Check sheet for the modelled part. Datum: model origin and axes. Units: mm. A direction names the side the tool comes from. Round coordinates to 2 decimals unless told otherwise and drop trailing zeros. Loops run counter-clockwise (first coordinate to the right, second up) from the corner with the lowest first, then second, coordinate; pieces in that order, holes last. Notation, with made-up numbers: (27.25, 27) - (41.25, 27) arc R18 cw to (41.25, 41) - close; hole circle Ø3 at (-9, -22.75). An arc over 180 degrees is marked (long way). Answer in a Markdown table with one row per item. Add a question column.
(1) Mould release check, pull along X, two halves, no side actions. Record for faces 3 (the cylindrical face through (10, 8, 2)), 4 (the flat face through (6.9, 2, -0.5)), 5 (the flat face through (14, 15, 2)): +X half, -X half, draft (parallel to the pull), parting line (faces both ways), or undercut.
(2) Gauge pin test, flat end, axial feed: pin 1 (4 mm diameter, centred on x = 6, y = 11, fed in from -Z). Record the tip position at first contact, or that the pin passes through.
(3) Thickness scan on line 1 along X through (y, z) = (12.5, 3.15); line 2 along Y through (x, z) = (7.75, -0.55); line 3 along Z through (x, y) = (6, 8.5). Record the ranges inside material, lowest first.
(4) Access from +Z, -Z, +X, -X, +Y, -Y to the whole of each face (thin tool, end or side, straight path). Record for faces 1 (the flat face through (6.9, 30, 3.5)), 2 (the flat face through (7, 9, 0)).
(5) Cross-section at A-A on y = 6. Enter the section's corners in (x, z), then the cut area to 3 significant figures.
(6) Cross-section at B-B on z = 3.4. Enter the section's corners in (x, y).
(7) Cross-section at C-C on z = 1.9. Enter the section's corners in (x, y).
from build123d import *

# Parameters (mm, degrees)
ESQUISSE1_W                = 14
ESQUISSE1_H                = 30
BASE_EXTRUSION_DEPTH       = 5
ESQUISSE2_W                = 4
ESQUISSE2_H                = 29
ENL_V_MAT_EXTRU_2_DEPTH    = 34.481338086
CONG_2_R                   = 3
ENL_V_MAT_EXTRU_3_DEPTH    = 20
R_P_TITION_LIN_AIRE1_COUNT = 14
R_P_TITION_LIN_AIRE1_PITCH = 1
ESQUISSE10_W               = 2
ESQUISSE10_H               = 3
ENL_V_MAT_EXTRU_17_DEPTH   = 20
ESQUISSE11_W               = 2
ESQUISSE11_H               = 2
BOSS_EXTRU_2_DEPTH         = 14
ESQUISSE12_R               = 2.5
ENL_V_MAT_EXTRU_18_DEPTH   = 34.346664001
ESQUISSE13_R               = 2.1
ENL_V_MAT_EXTRU_19_DEPTH   = 14


with BuildPart() as part:
    # Esquisse1 → Base-Extrusion (new body)
    with BuildSketch(Plane.XY):
        with Locations((7, 15)):
            Rectangle(ESQUISSE1_W, ESQUISSE1_H)
    extrude(amount=BASE_EXTRUSION_DEPTH)

    # Esquisse2 → Enlèv. mat.-Extru.2 (cut, through all)
    with BuildSketch(Plane(origin=(14, 0, 0), x_dir=(0, 0, -1), z_dir=(1, 0, 0))):
        with Locations((-6, 16.5)):
            Rectangle(ESQUISSE2_W, ESQUISSE2_H)
    extrude(amount=-ENL_V_MAT_EXTRU_2_DEPTH, mode=Mode.SUBTRACT)

    # Congé2
    cong_2_edges = [part.edges().sort_by_distance(p)[0] for p in [
        (7, 30, 0),
    ]]
    fillet(cong_2_edges, radius=CONG_2_R)

    # Esquisse3 → Enlèv. mat.-Extru.3 (cut)
    with BuildSketch(Plane(origin=(0, 30, 0), x_dir=(-1, 0, 0), z_dir=(0, 1, 0))):
        Polygon((-13.9, 0), (-13.1, 0), (-13.5, 0.4), align=None)
    enl_v_mat_extru_3 = extrude(amount=-ENL_V_MAT_EXTRU_3_DEPTH, mode=Mode.SUBTRACT)

    # Répétition linéaire1: Enlèv. mat.-Extru.3 ×14
    with Locations(*[(-i * R_P_TITION_LIN_AIRE1_PITCH, 0, 0) for i in range(1, R_P_TITION_LIN_AIRE1_COUNT)]):
        add(enl_v_mat_extru_3, mode=Mode.SUBTRACT)

    # Esquisse10 → Enlèv. mat.-Extru.17 (cut)
    with BuildSketch(Plane.ZY):
        with Locations((5, 0.5)):
            Rectangle(ESQUISSE10_W, ESQUISSE10_H)
    extrude(amount=-ENL_V_MAT_EXTRU_17_DEPTH, mode=Mode.SUBTRACT)

    # Esquisse11 → Boss.-Extru.2 (add)
    with BuildSketch(Plane.ZY):
        with Locations((0, 1)):
            Rectangle(ESQUISSE11_W, ESQUISSE11_H)
    extrude(amount=-BOSS_EXTRU_2_DEPTH)

    # Esquisse12 → Enlèv. mat.-Extru.18 (cut, through all)
    with BuildSketch(Plane(origin=(0, 0, 0), x_dir=(-1, 0, 0), z_dir=(0, 0, -1))):
        with Locations((-8.5, 6)):
            Circle(ESQUISSE12_R)
    extrude(amount=-ENL_V_MAT_EXTRU_18_DEPTH, mode=Mode.SUBTRACT)

    # Esquisse13 → Enlèv. mat.-Extru.19 (cut)
    with BuildSketch(Plane(origin=(0, 0, 0), x_dir=(-1, 0, 0), z_dir=(0, 0, -1))):
        with Locations((-5.9, 12.5)):
            Circle(ESQUISSE13_R)
    extrude(amount=-ENL_V_MAT_EXTRU_19_DEPTH, mode=Mode.SUBTRACT)


solid = part.part
Answers:
| question | item | result |
|---|---|---|
| 1 | face 3 | undercut |
| 1 | face 4 | draft |
| 1 | face 5 | +X half |
| 2 | pin 1 | stops at z = 0 |
| 3 | line 1 | x = 0 to 3.8, 8 to 14 |
| 3 | line 2 | y = 0 to 2 |
| 3 | line 3 | z = 0 to 4 |
| 4 | face 1 | +Z, -Z, +X, -X, +Y |
| 4 | face 2 | -Z, +X, -X, +Y |
| 5 | outline | (0, 0) - (6, 0) - (6, 4) - (0, 4) - close; (11, 0) - (14, 0) - (14, 4) - (11, 4) - close |
| 5 | area | 36.0 mm^2 |
| 6 | outline | (0, 0) - (14, 0) - (14, 30) - (0, 30) - close; hole circle Ø4.2 at (5.9, 12.5); hole circle Ø5 at (8.5, 6) |
| 7 | outline | (0, 0) - (14, 0) - (14, 29.79) - (0, 29.79) - close; hole circle Ø4.2 at (5.9, 12.5); hole circle Ø5 at (8.5, 6) |
